The model under review builds one solid part; all positions refer to its coordinate system, in mm. A direction names the side the tool comes from. Coordinates: 2 decimals unless noted, no trailing zeros. Order: outer loops, then holes, each group sorted by start corner. A loop starts at its lowest first (then second) coordinate and runs counter-clockwise, first axis right, second up. Notation, with made-up numbers: M 76,-27 L 116,-27 A3 ccw 116,-23 Z; hole C 64.25,4 d10. An arc over 180 degrees is marked long. One line per item, written item: value.
Autodesk Inventor part; units mm, degrees
ref_plane "YZ Plane" through (0, 0, 0) normal (1, 0, 0) x (0, 1, 0)
ref_plane "XZ Plane" through (0, 0, 0) normal (0, 1, 0) x (-1, 0, 0)
ref_plane "XY Plane" through (0, 0, 0) normal (0, 0, 1) x (1, 0, 0)
sketch "Sketch1" plane through (0, 0, 0) normal (0, 1, 0) x (-1, 0, 0)
  line L0 (0, 18.5) -> (4, 18.5)
  line L1 (4, 18.5) -> (4, 14.5)
  line L2 (4, 14.5) -> (0, 14.5)
  line L3 (0, 14.5) -> (0, 18.5)
  line L4 (4, -14.5) -> (0, -14.5)
  line L5 (0, -14.5) -> (0, -18.5)
  line L6 (0, -18.5) -> (4, -18.5)
  line L7 (4, -18.5) -> (4, -14.5)
  line L8 (4, 14.5) -> (4, -14.5) construction
  point P0 (0, 0)
  point P1 (4, 0)
  dimension "d0" = 37
  dimension "d1" = 4
extrude "Extrusion1" add sketch "Sketch1" along normal blind 2
sketch "Sketch2" plane through (0, 2, 0) normal (0, 1, 0) x (1, 0, 0)
  line L0 (-4, -14.5) -> (-4, -18.5)
  line L1 (0, 14.5) -> (0, 18.5)
  line L2 (-4, -16.5) -> (0, -16.5)
  line L3 (0, -16.5) -> (0, 16.5)
  line L4 (0, 16.5) -> (-4, 16.5)
  line L5 (-4, 16.5) -> (-4, -16.5)
  line L6 (0, -14.5) -> (-4, -14.5)
  line L7 (-4, 14.5) -> (0, 14.5)
  point P0 (0, 0)
  dimension "d4" = 2
  dimension "d5" = 2
extrude "Extrusion2" add sketch "Sketch2" along normal blind 2 contours L6 L3 L2 L0 | L5 L4 L1 L7
sketch "Sketch3" plane through (0, 4, 0) normal (0, 1, 0) x (1, 0, 0)
  line L0 (-4, -16.5) -> (0, -16.5)
  line L1 (0, 16.5) -> (-4, 16.5)
  line L2 (0, -16.5) -> (-4, -16.5)
  line L3 (-4, -16.5) -> (-4, 16.5)
  line L4 (-4, 16.5) -> (0, 16.5)
  line L5 (0, 16.5) -> (0, -16.5)
  point P0 (0, 0)
extrude "Extrusion3" add sketch "Sketch3" along normal blind 2
fillet "Fillet3" radius 1 9 edges at (-2, 2, 16.5) (-2, 2, 18.5) (-2, 2, -16.5) (-2, 0, 14.5) (-2, 0, -14.5) (-2, 4, -14.5) (-2, 4, 14.5) (-2, 6, -16.5) (-2, 6, 16.5)
fillet "Fillet4" radius 1 1 edges at (-2, 2, -18.5)
properties part number "screen_support"
(1) We need section C-C, the plane z = -8.5. State the section outline as (x, y) points.
Geometry results:
outline: M -4,4 L 0,4 L 0,6 L -4,6 Z
(2) Mouldability with a two-part tool opening along Z and no side actions: class faces 1 (the cylindrical face through (-2.028, 5.715, -16.199)), 2 (the cylindrical face through (-2.028, 3.699, 14.215)), 3 (the flat face through (0, 4.3, 3.9)) as +Z half, -Z half, draft (parallel to the pull), parting line (faces both ways), or undercut.
Geometry results:
face 1: -Z half
face 2: undercut
face 3: draft
(3) For L1, parallel to Z at x = -1.45, y = 3; L2, parallel to Y at x = -1.75, z = -12.5; L3, parallel to Z at x = -2.6, y = 3.85, list the stretches that pass through material, from the lowest coordinate up.
Geometry results:
L1: z = -16.5 to -14.5, 14.5 to 16.5
L2: y = 4 to 6
L3: z = -16.5 to -14.03, 14.03 to 16.5
(4) Insertion check: pin 1 Ø3 at (y, z) = (2, -12.5) entering from +X; pin 2 Ø2 at (x, y) = (-1.5, 3.5) entering from +Z; pin 3 Ø0.6 at (x, y) = (-1.5, 1.5) entering from -Z; pin 4 Ø0.6 at (x, y) = (-1.5, 1.5) entering from +Z. Each pin has a flat end and moves straight along its axis. Give the tip position at first contact, or say it passes through.
Geometry results:
pin 1: passes through
pin 2: stops at z = 16.63
pin 3: stops at z = -18.48
pin 4: stops at z = 18.48
(5) We need section D-D, the plane y = 4.5. State the section outline as (x, z) points, plus the area to 3 significant figures.
Geometry results:
outline: M -4,-16.5 L 0,-16.5 L 0,16.5 L -4,16.5 Z
area: 132 mm2
(6) We need section B-B, the plane y = 2.65. State the section outline as (x, z) points.
Geometry results:
outline: M -4,-16.56 L 0,-16.56 L 0,-14.5 L -4,-14.5 Z; M -4,14.5 L 0,14.5 L 0,16.56 L -4,16.56 Z
(7) Tool access review of faces 4 (the flat face through (-2, 4, 16.5)), 5 (the cylindrical face through (-1.972, 3.699, -14.215)), 6 (the cylindrical face through (-2.028, 2.285, -16.801)): name each direction out of +Z, -Z, +X, -X, +Y, -Y from which nothing blocks a thin tool from reaching the whole face with its end or side.
Geometry results:
face 4: +Z, +X, -X, +Y
face 5: +X, -X, -Y
face 6: -Z, +X, -X, +Y
